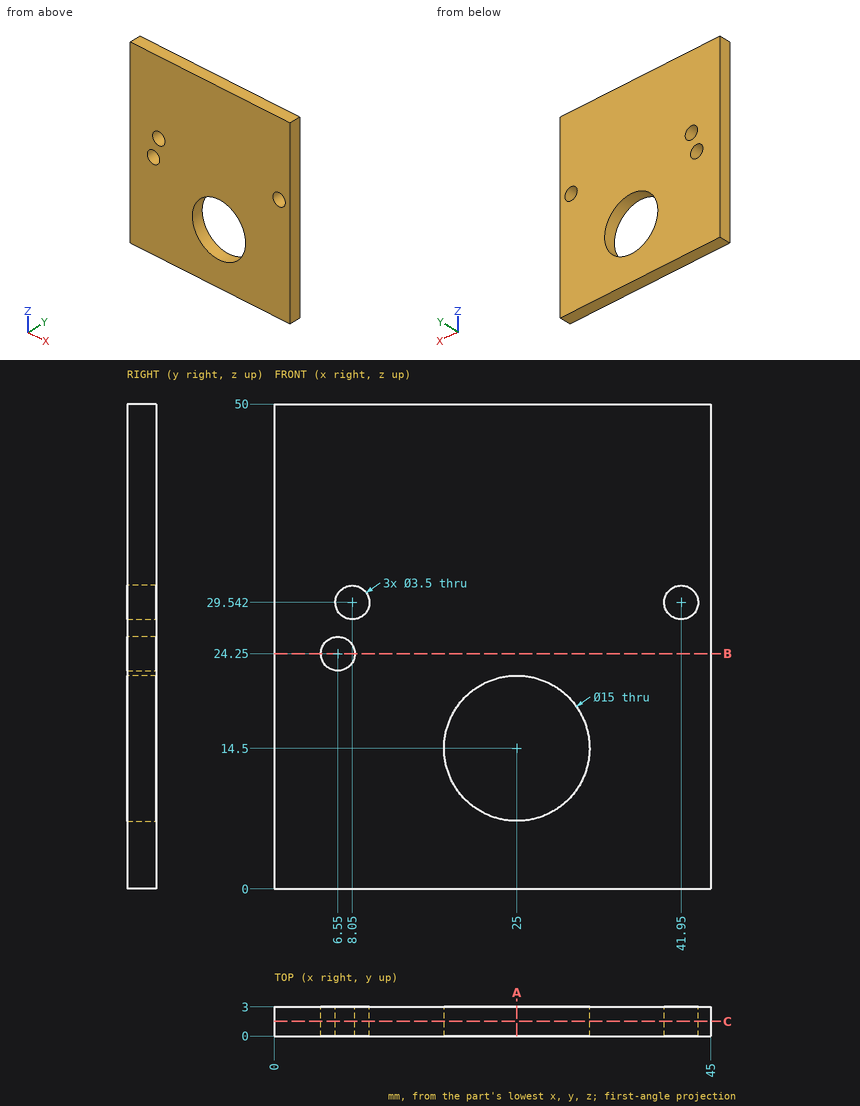
The figure shows three views and two pictorial views of one solid part (mm, origin at its lowest corner). Answer the questions. Give positions to 0.01 mm unless a question says otherwise; leave off trailing zeros. Write each loop counter-clockwise with the first axis right and the second up, starting at its lowest first coordinate (ties: lowest second). Pieces come first, ordered by that corner, then holes. Notation, with made-up numbers: (38, 71.25) - (97, 71.25) arc R24 cw to (97, 81.25) - close; hole circle Ø11 at (3.25, 3.25). An arc over 180 degrees is marked (long way). Use one line per item in the form item = value. Start each with the question number.
1) Consider line 1 along X through (y, z) = (0.75, 14.5); line 2 along X through (y, z) = (1.85, 24.25); line 3 along Z through (x, y) = (28, 1.1) (1 decimal). Determine where each line is inside the solid, lowest interval first. Write a range as from..to.
2) Find section A-A on x = 25. Determine the outline of the cut face in (y, z), plus the area to 3 significant figures.
3) A flat-ended cylindrical pin translates along its axis: pin 1 Ø12 at (x, z) = (25, 14.5) entering from -Y. Find the tip coordinate at first contact, or state that the pin passes through.
4) Find section C-C on y = 1.5. Determine the outline of the cut face in (x, z).
5) Find section B-B on z = 24.25. Determine the outline of the cut face in (x, y).
Geometry results:
q1.line_1 = 0..17.5, 32.5..45
q1.line_2 = 0..4.8, 8.3..45
q1.line_3 = 0..7.6, 21.4..50
q2.outline = (0, 0) - (3, 0) - (3, 7) - (0, 7) - close; (0, 22) - (3, 22) - (3, 50) - (0, 50) - close
q2.area = 105 mm2
q3.pin_1 = through
q4.outline = (0, 0) - (45, 0) - (45, 50) - (0, 50) - close; hole circle Ø3.5 at (6.55, 24.25); hole circle Ø3.5 at (8.05, 29.54); hole circle Ø15 at (25, 14.5); hole circle Ø3.5 at (41.95, 29.54)
q5.outline = (0, 0) - (4.8, 0) - (4.8, 3) - (0, 3) - close; (8.3, 0) - (45, 0) - (45, 3) - (8.3, 3) - close
